Autodesk Inventor part; units mm, degrees
ref_plane "YZ Plane" through (0, 0, 0) normal (1, 0, 0) x (0, 1, 0)
ref_plane "XZ Plane" through (0, 0, 0) normal (0, 1, 0) x (-1, 0, 0)
ref_plane "XY Plane" through (0, 0, 0) normal (0, 0, 1) x (1, 0, 0)
sketch "Sketch1" plane through (0, 0, 0) normal (0, 1, 0) x (-1, 0, 0)
  line L0 (0, 0) -> (-130, 0)
  line L1 (-130, 0) -> (-130, -100)
  line L2 (-130, -100) -> (0, -100)
  line L3 (0, -100) -> (0, 0)
  dimension "d0" = 130
  dimension "d1" = 100
extrude "Extrusion1" add sketch "Sketch1" along normal blind 10
sketch "Sketch2" plane through (0, 10, 0) normal (0, 1, 0) x (1, 0, 0)
  line L0 (10, 25) -> (120, 25)
  line L1 (120, 25) -> (120, 75)
  line L2 (120, 75) -> (10, 75)
  line L3 (10, 75) -> (10, 25)
  line L4 (130, 100) -> (0, 100)
  line L5 (130, 0) -> (130, 100)
  line L6 (0, 100) -> (0, 0)
  line L7 (0, 0) -> (130, 0)
  dimension "d4" = 25
  dimension "d5" = 10
  dimension "d6" = 10
  dimension "d7" = 25
extrude "Extrusion2" add sketch "Sketch2" along normal blind 40
sketch "Sketch3" plane through (0, 50, 0) normal (0, 1, 0) x (1, 0, 0)
  circle A0 centre (10, 90) radius 3
  line L0 (130, 100) -> (0, 100)
  line L1 (0, 100) -> (0, 0)
  line L2 (130, 0) -> (130, 100)
  line L3 (130, 100) -> (0, 100)
  line L4 (65, 100) -> (65, 0)
  line L5 (0, 0) -> (130, 0)
  line L6 (0, 100) -> (0, 0)
  line L7 (0, 50) -> (130, 50)
  circle A1 centre (120, 90) radius 3
  circle A2 centre (10, 10) radius 3
  line L8 (130, 0) -> (0, 0)
  line L9 (130, 0) -> (0, 0)
  circle A3 centre (120, 10) radius 3
  dimension "d10" = 6
  dimension "d11" = 10
  dimension "d12" = 10
extrude "Extrusion3" add sketch "Sketch3" along normal blind 40 contours A0 | A1 | A2 | A3
properties part number "bottom"
Read the model definition and answer for the solid it produces. Units are mm, in the model's axes. A direction names the side the tool comes from. Give positions to 0.01 mm unless a question says otherwise; leave off trailing zeros. Loops run counter-clockwise (first coordinate to the right, second up) from the corner with the lowest first, then second, coordinate; pieces in that order, holes last. Notation, with made-up numbers: (48, 18.25) - (73, 18.25) arc R8 ccw to (73, 24.25) - close; hole circle Ø1 at (-22.5, 69.5). An arc over 180 degrees is marked (long way). Answer as CSV lines item,"result". Start each with the question number.
1) Find section B-B (x = 31). Write down the section's boundary in (y, z), then the cut area to 3 significant figures.
2) Find section D-D (z = -90). Write down the section's boundary in (x, y).
3) Which of the six approach directions +Z, -Z, +X, -X, +Y, -Y give full straight-line access (tool end or side, diameter ignored) to faces 1 (the face through (121.384, 69.72, -92.662)), 2 (the face through (66, 25, -100))?
4) Determine the mould class of faces 3 (the face through (11.61, 69.72, -7.47)), 4 (the face through (0, 25, -51)), 5 (the face through (66, 0, -49)) for opening direction X: released by +X, released by -X, zero draft, split by the parting line, or undercut.
5) Each of these flat-tipped pins is pushed along its axis until it touches: pin 1 Ø5 at (x, y) = (75, 54.5) entering from +Z; pin 2 Ø1.5 at (x, z) = (116, -69) entering from +Y. Where does it stop, or does it pass through?
6) Find section A-A (z = -52.5). Write down the section's boundary in (x, y), then the cut area to 3 significant figures.
7) Straight lines are drawn through the part: L1, parallel to Z at x = 65.5, y = 29.5; L2, parallel to X at y = 23, z = -39; L3, parallel to Z at x = 120, y = 51.5. For each, find the intervals that lie inside material, in ascending order. Write a range as from..to.
8) Find section C-C (y = 77). Write down the section's boundary in (x, z).
Findings below:
1,outline,"(0, -100) - (50, -100) - (50, -75) - (10, -75) - (10, -25) - (50, -25) - (50, 0) - (0, 0) - close"
1,area,"3,000 mm^2"
2,outline,"(0, 0) - (130, 0) - (130, 50) - (123, 50) - (123, 90) - (117, 90) - (117, 50) - (13, 50) - (13, 90) - (7, 90) - (7, 50) - (0, 50) - close"
3,face 1,"+Y"
3,face 2,"-Z, +X, -X, +Y, -Y"
4,face 3,"undercut"
4,face 4,"released by -X"
4,face 5,"zero draft"
5,pin 1,"through"
5,pin 2,"y = 10"
6,outline,"(0, 0) - (130, 0) - (130, 50) - (120, 50) - (120, 10) - (10, 10) - (10, 50) - (0, 50) - close"
6,area,"2,100 mm^2"
7,L1,"-100..-75, -25..0"
7,L2,"0..10, 120..130"
7,L3,"-93..-87, -13..-7"
8,outline,"circle Ø6 at (10, -90); circle Ø6 at (10, -10); circle Ø6 at (120, -90); circle Ø6 at (120, -10)"
